Part model, mm, in its own coordinate system. A direction names the side the tool comes from. Coordinates: 2 decimals unless noted, no trailing zeros. Loops run counter-clockwise (first coordinate to the right, second up) from the corner with the lowest first, then second, coordinate; pieces in that order, holes last. Notation, with made-up numbers: (57, 27.25) - (83, 27.25) arc R26 cw to (83, 60.25) - close; hole circle Ø6 at (33.5, -27). An arc over 180 degrees is marked (long way). Answer as CSV lines item,"result".
from build123d import *

# Parameters (mm, degrees)
F0_W     = 203.2
F0_H     = 127
F1_DEPTH = 127
F3_DEPTH = 76.2
F4_SIZE2 = 101.6
F4_SIZE  = 76.2
F5_R     = 5.08
F6_R     = 15.24
F7_DEPTH = 50.8
F8_R     = 15.24
F9_DEPTH = 127


with BuildPart() as f1:
    # F0 (on Front) → F1 (new body)
    with BuildSketch(Plane.XZ):
        with Locations((-1.3009174736, 0.3703823313)):
            Rectangle(F0_W, F0_H)
    extrude(amount=F1_DEPTH)

    # F2 (on face) → F3 (cut)
    with BuildSketch(Plane.XZ.offset(127)):
        Polygon((-39.4009174736, 0), (-39.4009174736, -63.1296176687), (100.2990825264, -63.1296176687), (100.2990825264, 63.8703823313), (-1.3009174736, 63.8703823313), (-1.3009174736, 0), align=None)
    extrude(amount=-F3_DEPTH, mode=Mode.SUBTRACT)

    # F4
    f4_edges = [f1.edges().sort_by_distance(p)[0] for p in [
        (100.299083, -25.4, 63.870382),
    ]]
    f4_side = f1.faces().sort_by_distance((-23.072346, -52.614286, 63.870382))[0]
    chamfer(f4_edges, length=F4_SIZE, length2=F4_SIZE2, reference=f4_side)

    # F5
    f5_edges = [f1.edges().sort_by_distance(p)[0] for p in [
        (11.399083, -50.8, 63.870382),
        (-1.300917, -88.9, 63.870382),
        (-52.100917, -127, 63.870382),
        (100.299083, -50.8, -50.429618),
        (62.199083, -50.8, 13.070382),
        (30.449083, -50.8, -63.129618),
        (-39.400917, -50.8, -31.564809),
        (-1.300917, -50.8, 31.935191),
        (-20.350917, -50.8, 0),
        (-1.300917, -127, 31.935191),
        (-1.300917, -88.9, 0),
        (-39.400917, -127, -31.564809),
        (100.299083, -25.4, -63.129618),
        (-71.150917, -127, -63.129618),
        (-39.400917, 0, 63.870382),
        (62.199083, 0, 13.070382),
        (-102.900917, -63.5, 63.870382),
        (-102.900917, -127, 0.370382),
        (-102.900917, 0, 0.370382),
        (-39.400917, -88.9, -63.129618),
    ]]
    fillet(f5_edges, radius=F5_R)

    # F6 (on face) → F7 (cut, through all)
    with BuildSketch(Plane.XZ.offset(50.8)):
        with Locations((29.1790825264, -17.4096176687)):
            Circle(F6_R)
    extrude(amount=-F7_DEPTH, mode=Mode.SUBTRACT)

    # F8 (on face) → F9 (cut, through all)
    with BuildSketch(Plane.XY.offset(63.8703823313)):
        with Locations((-56.2786398957, -80.1086086328)):
            Circle(F8_R)
    extrude(amount=-F9_DEPTH, mode=Mode.SUBTRACT)


solid = f1.part
Q1. Which spindle directions (+Z, -Z, +X, -X, +Y, -Y) get a long thin tool onto all of the face, cutting with end or side? Do faces 1 (the face through (-2.829, -88.438, 62.422)), 2 (the face through (63, -25, 12)), 3 (the face through (-2.75, -90.942, 1.528)). Say none if no direction does.
Results:
face 1,"+Z, +X, -Y"
face 2,"+Z, +X, +Y, -Y"
face 3,"-Z, +X, -Y"
Q2. Flat gauge pins, fed straight in: pin 1 (2 mm diameter, centred on x = -9, y = -69.5, fed in from -Z); pin 2 (1 mm diameter, centred on y = -59, z = -7, fed in from +X). Where does each tip first touch, or does it go through?
Results:
pin 1,"stops at z = 0"
pin 2,"stops at x = -39.4"
Q3. Wall check: L1, parallel to Y at x = -55, z = -48; L2, parallel to X at y = -96.5, z = -51; L3, parallel to Z at x = -19.5, y = -62.5. Give the ranges that are in metal, low to high.
Results:
L1,"y = -127 to -95.29, -64.92 to 0"
L2,"x = -102.9 to -39.4"
L3,"z = 0 to 63.87"
Q4. Saw through at B-B (x = -57). Give the cut face in (y, z), then the cut area to 3 significant figures.
Results:
outline,"(-127, -58.05) arc R5.08 ccw to (-121.92, -63.13) - (-95.33, -63.13) - (-95.33, 63.87) - (-121.92, 63.87) arc R5.08 ccw to (-127, 58.79) - close; (-64.89, -63.13) - (0, -63.13) - (0, 58.79) arc R5.08 ccw to (-5.08, 63.87) - (-64.89, 63.87) - close"
area,"12,200 mm^2"
Q5. Saw through at D-D (z = -50). Give the cut face in (x, y).
Results:
outline,"(-102.9, -121.92) arc R5.08 ccw to (-97.82, -127) - (-44.48, -127) arc R5.08 ccw to (-39.4, -121.92) - (-39.4, -55.88) arc R5.08 cw to (-34.32, -50.8) - (95.22, -50.8) arc R5.08 ccw to (100.3, -45.72) - (100.3, 0) - (-97.82, 0) arc R5.08 ccw to (-102.9, -5.08) - close; hole circle Ø30.48 at (-56.28, -80.11)"
Q6. Saw through at C-C (z = -27.5). Count the separate pieces of the cut face and the enclosed holes in it, then the cut area to 3 significant figures.
Results:
separate pieces,"2"
enclosed holes,"1"
area,"12,900 mm^2"
Q7. Saw through at A-A (y = -108). Give the cut face in (x, z).
Results:
outline,"(-102.9, -63.13) - (-44.48, -63.13) arc R5.08 ccw to (-39.4, -58.05) - (-39.4, 0) - (-6.38, 0) arc R5.08 ccw to (-1.3, 5.08) - (-1.3, 58.79) arc R5.08 ccw to (-6.38, 63.87) - (-97.82, 63.87) arc R5.08 ccw to (-102.9, 58.79) - close"
